Input: part model. Units: mm. Frame: model coordinates. A direction names the side the tool comes from. Coordinates: 2 decimals unless noted, no trailing zeros. Loops run counter-clockwise (first coordinate to the right, second up) from the corner with the lowest first, then second, coordinate; pieces in that order, holes last.
```python
from build123d import *

# Parameters (mm, degrees)
F0_W      = 116.4761967957
F0_H      = 82.8055683523
F1_DEPTH  = 37
F2_R      = 13.9038489757
F3_DEPTH  = 14.2
F6_R      = 10.3135851835
F7_DEPTH  = 11.5
F8_R      = 8.6398790052
F9_DEPTH  = 33.5
F10_R     = 21.7279220614
F11_R     = 29.2119841047
F12_W     = 11.8597049732
F12_H     = 3.4746369347
F13_DEPTH = 25


# Not quite as in the source:
# - the program builds the solid bodies; features that only make, move or delete a surface that nothing else refers to are left out


with BuildPart() as f1:
    # F0 (on Top) → F1 (new body)
    with BuildSketch(Plane.XY):
        with Locations((0.5078110844, -10.3384470567)):
            Rectangle(F0_W, F0_H)
    extrude(amount=F1_DEPTH)

    # F2 (on face) → F3 (join)
    with BuildSketch(Plane.XY.offset(37)):
        with Locations((33.5578107329, -14.6564913073)):
            Circle(F2_R)
    extrude(amount=F3_DEPTH)

    # F6 (on face) → F7 (join)
    with BuildSketch(Plane.XY.offset(51.2)):
        with Locations((33.5578107329, -14.6564913073)):
            Circle(F6_R)
    extrude(amount=F7_DEPTH)

    # F8 (on face) → F9 (cut)
    with BuildSketch(Plane.XY.offset(62.7)):
        with Locations((33.5578107329, -14.6564913073)):
            Circle(F8_R)
    extrude(amount=-F9_DEPTH, mode=Mode.SUBTRACT)

    # F10
    f10_edges = [f1.edges().sort_by_distance(p)[0] for p in [
        (58.745909, 31.064337, 18.5),
    ]]
    fillet(f10_edges, radius=F10_R)

    # F11
    f11_edges = [f1.edges().sort_by_distance(p)[0] for p in [
        (-57.730287, -51.741231, 18.5),
    ]]
    fillet(f11_edges, radius=F11_R)

    # F12 (on face) → F13 (cut)
    with BuildSketch(Plane.XY.offset(37)):
        with Locations((-2.380865044, 17.2674548812)):
            Rectangle(F12_W, F12_H)
    extrude(amount=-F13_DEPTH, mode=Mode.SUBTRACT)


solid = f1.part
```
Item 1: Line query: L1, parallel to X at y = -15, z = 51.5; L2, parallel to Z at x = -50, y = -41.5; L3, parallel to X at y = -18.5, z = 55.5. Output: solid intervals per line, ascending.
Result:
L1: x = 23.25 to 24.92, 42.19 to 43.87
L2: z = 0 to 37
L3: x = 23.99 to 25.82, 41.3 to 43.13
Item 2: Contact query for flat-ended pins moving along their axis: P1, Ø12, axis at x = -12, y = 10, coming from the +Z side; P2, Ø3, axis at y = 17, z = 30.5, coming from the +X side; P3, Ø8.5, axis at x = 32.5, y = -17, coming from the +Z side. Output: stop coordinate, or through.
Result:
P1: stops at z = 37
P2: stops at x = 57.85
P3: stops at z = 29.2
Item 3: Mould query, pull axis X, two halves, no side actions, for faces 1 (the face through (-49.4, -42.957, 18.759)), 2 (the face through (0, -10, 0)), 3 (the face through (-2, 19.005, 25)). Classes: +X half, -X half, draft (parallel to the pull), parting line (faces both ways), or undercut.
Result:
face 1: -X half
face 2: draft
face 3: undercut
Item 4: Section query D-D (x = 40.5). Output: boundary loops of the cut face in (y, z), then the cut area to 3 significant figures.
Result:
outline: (-51.74, 0) - (30.78, 0) - (30.78, 37) - (-2.61, 37) - (-2.61, 51.2) - (-7.03, 51.2) - (-7.03, 62.7) - (-9.51, 62.7) - (-9.51, 29.2) - (-19.8, 29.2) - (-19.8, 62.7) - (-22.28, 62.7) - (-22.28, 51.2) - (-26.7, 51.2) - (-26.7, 37) - (-51.74, 37) - close
area: 3,230 mm2
Item 5: Section query A-A (z = 27). Output: boundary loops of the cut face in (x, y).
Result:
outline: (-57.73, -22.53) arc R29.21 ccw to (-28.52, -51.74) - (58.75, -51.74) - (58.75, 9.34) arc R21.73 ccw to (37.02, 31.06) - (-57.73, 31.06) - close; hole (-8.31, 15.53) - (3.55, 15.53) - (3.55, 19) - (-8.31, 19) - close
Item 6: Section query B-B (y = -3). Output: boundary loops of the cut face in (x, z), then the cut area to 3 significant figures.
Result:
outline: (-57.73, 0) - (58.75, 0) - (58.75, 37) - (41.14, 37) - (41.14, 51.2) - (25.98, 51.2) - (25.98, 37) - (-57.73, 37) - close
area: 4,520 mm2
Item 7: Section query C-C (x = 11). Output: boundary loops of the cut face in (y, z).
Result:
outline: (-51.74, 0) - (31.06, 0) - (31.06, 37) - (-51.74, 37) - close
Item 8: Reachability of faces 4 (the face through (-8.311, 17, 25)), 5 (the face through (52.21, 24.87, 18.76)) from +Z, -Z, +X, -X, +Y, -Y: full face, straight path, thin tool, end or side. Return the list, or none.
Result:
face 4: +Z
face 5: +Z, -Z, +X, +Y
